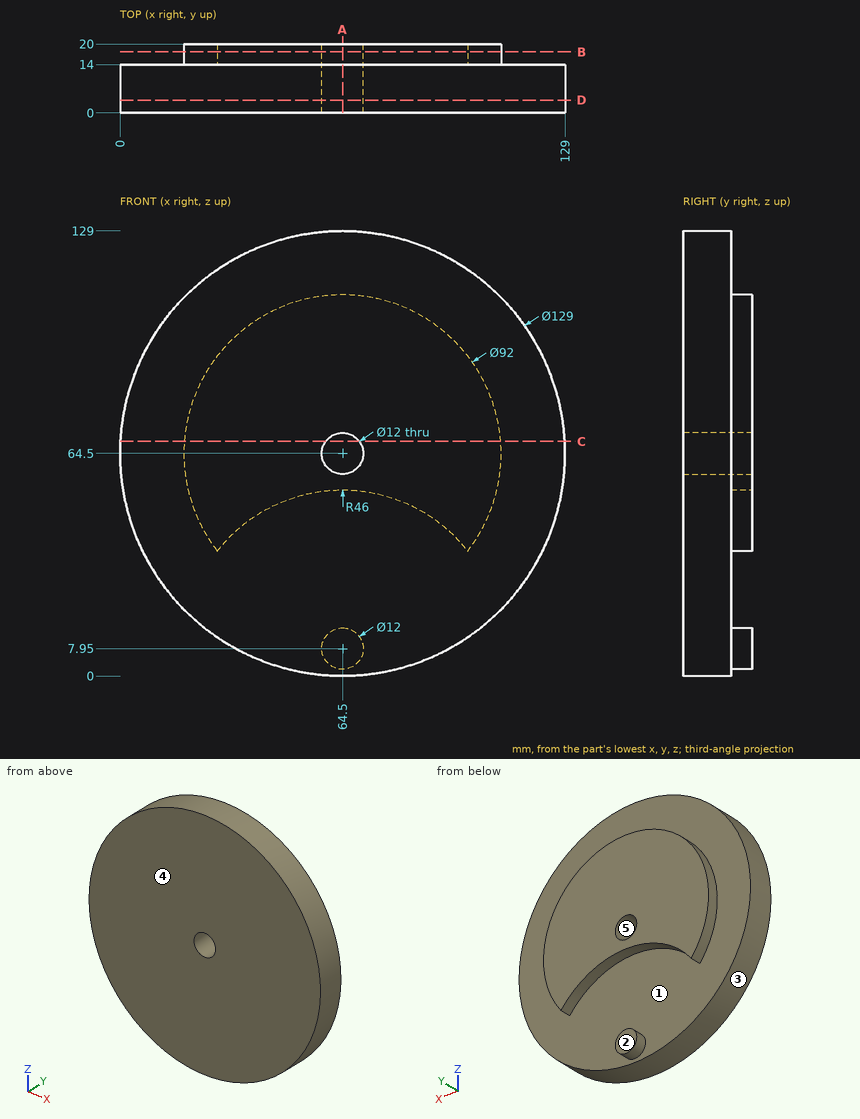
Check sheet for the drawn part. Datum: minimum x, y, z corner. Units: mm. A direction names the side the tool comes from. Give positions to 0.01 mm unless a question says otherwise; leave off trailing zeros. Loops run counter-clockwise (first coordinate to the right, second up) from the corner with the lowest first, then second, coordinate; pieces in that order, holes last. Notation, with made-up numbers: M 51.25,88 L 69.25,88 A8 cw 69.25,100 Z; hole C 48,52.25 d9. An arc over 180 degrees is marked long. Answer as CSV lines item,"result".
Item 1: Sectioned sample at C-C, the plane z = 68. Enter the section's corners in (x, y), then the cut area to 3 significant figures.
Reply:
outline,"M 0.1,0 L 59.63,0 L 59.63,20 L 18.63,20 L 18.63,14 L 0.1,14 Z; M 69.37,0 L 128.9,0 L 128.9,14 L 110.37,14 L 110.37,20 L 69.37,20 Z"
area,"2,160 mm^2"
Item 2: Sectioned sample at D-D, the plane y = 3.75. Enter the section's corners in (x, z), then the cut area to 3 significant figures.
Reply:
outline,"C 64.5,64.5 d129; hole C 64.5,64.5 d12"
area,"13,000 mm^2"
Item 3: Scan lines: L1, parallel to X at y = 9.5, z = 64.5; L2, parallel to Y at x = 111, z = 50.5; L3, parallel to X at y = 12, z = 10.5. Record each from-to range of solid material in increasing order.
Reply:
L1,"0 to 58.5, 70.5 to 129"
L2,"0 to 14"
L3,"29.23 to 99.77"
Item 4: Depth check by flat-ended pin: pin 1 Ø12 at (x, y) = (78, 11) entering from -Z; pin 2 Ø8 at (y, z) = (7, 68.5) entering from -X; pin 3 Ø1 at (x, z) = (63, 68.5) entering from +Y; pin 4 Ø4 at (y, z) = (3.5, 110.5) entering from +X. Enter the tip coordinate at first touch or a pass-through.
Reply:
pin 1,"z = 0.44"
pin 2,"x = 0"
pin 3,"through"
pin 4,"x = 111.66"
Item 5: Sectioned sample at A-A, the plane x = 64.5. Enter the section's corners in (y, z), then the cut area to 3 significant figures.
Reply:
outline,"M 0,0 L 14,0 L 14,1.95 L 20,1.95 L 20,13.95 L 14,13.95 L 14,53.95 L 20,53.95 L 20,58.5 L 0,58.5 Z; M 0,70.5 L 20,70.5 L 20,110.5 L 14,110.5 L 14,129 L 0,129 Z"
area,"1,980 mm^2"
Item 6: Set-up check for the marked faces 1 and 2: record each of +Z, -Z, +X, -X, +Y, -Y from which the full face is reachable in a straight line by a thin tool's end or side.
Reply:
face 1,"+Y"
face 2,"+Z, -Z, +X, -X, +Y"
Item 7: Draft check along X on the marked faces 3, 4 and 5. Enter one of: pulls with the +X half, pulls with the -X half, needs draft (parallel to the pull), parting line crosses it, or undercut.
Reply:
face 3,"parting line crosses it"
face 4,"needs draft"
face 5,"undercut"
Item 8: Sectioned sample at B-B, the plane y = 17.75. Enter the section's corners in (x, z) (3 decimals), then the cut area to 3 significant figures.
Reply:
outline,"M 28.216,36.225 A46 cw 100.784,36.225 A46 ccw long Z; C 64.5,7.95 d12; hole C 64.5,64.5 d12"
area,"4,850 mm^2"
